Print and shaded views of the part. All mm, measured from the part's lowest x, y and z. Round coordinates to 2 decimals unless told otherwise and drop trailing zeros. Write each loop counter-clockwise with the first axis right and the second up, starting at its lowest first coordinate (ties: lowest second). Pieces come first, ordered by that corner, then holes. Notation, with made-up numbers: M -29,27.25 L 0,27.25 A27 ccw 0,47.25 Z; hole C -17.5,-25.5 d1. An arc over 180 degrees is marked long. Write item = value, one per line.
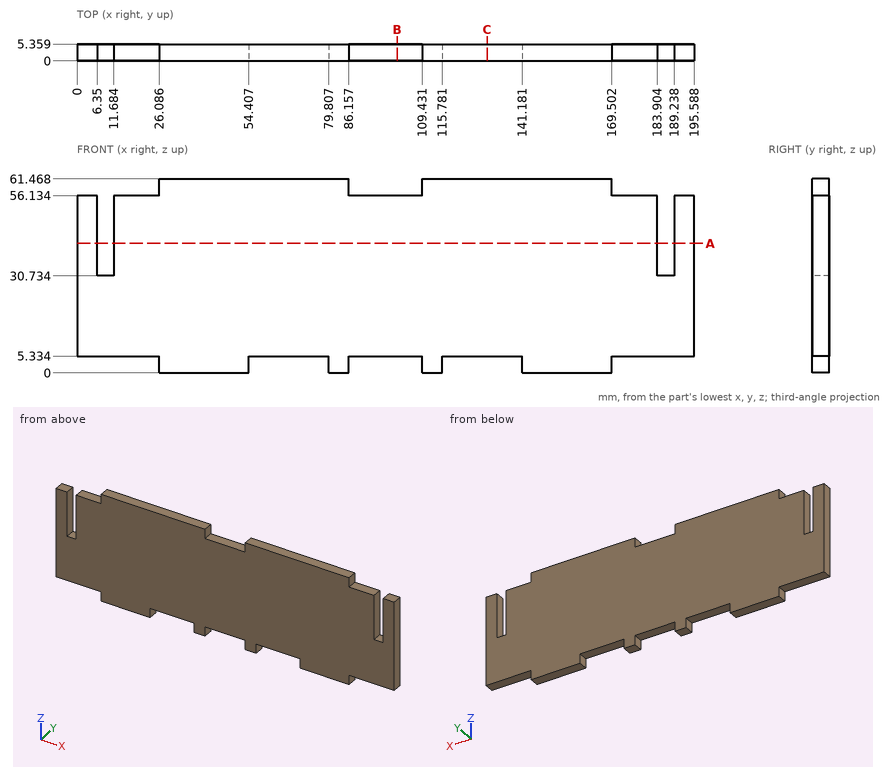
1. Band-saw the part on A-A (z = 41). List the corners of the cut face in (x, y), plus the area to 3 significant figures.
Responses:
outline = M 0,0 L 6.35,0 L 6.35,5.36 L 0,5.36 Z; M 11.68,0 L 183.9,0 L 183.9,5.36 L 11.68,5.36 Z; M 189.24,0 L 195.59,0 L 195.59,5.36 L 189.24,5.36 Z
area = 991 mm²
2. Band-saw the part on C-C (x = 130). List the corners of the cut face in (y, z), plus the area to 3 significant figures.
Responses:
outline = M 0,5.33 L 5.36,5.33 L 5.36,61.47 L 0,61.47 Z
area = 301 mm²
3. Probe probe 1 along X at (y, z) = (4.95, 50.5); probe 2 along Z at (x, y) = (137.5, 2.1); probe 3 along Z at (x, y) = (100, 2.6). List the from-to ranges inside material, lowest first.
Responses:
probe_1 = 0 to 6.35, 11.68 to 183.9, 189.24 to 195.59
probe_2 = 5.33 to 61.47
probe_3 = 5.33 to 56.13
4. Flat gauge pins, fed straight in: pin 1 (1.6 mm diameter, centred on x = 178.5, y = 2.5, fed in from +Z); pin 2 (2.5 mm diameter, centred on y = 3, z = 1.5, fed in from +X); pin 3 (2.5 mm diameter, centred on y = 3.5, z = 58, fed in from -X). Where does each tip first touch, or does it go through?
Responses:
pin_1 = 56.13
pin_2 = 169.5
pin_3 = 26.09
5. Band-saw the part on B-B (x = 101.5). List the corners of the cut face in (y, z).
Responses:
outline = M 0,5.33 L 5.36,5.33 L 5.36,56.13 L 0,56.13 Z
